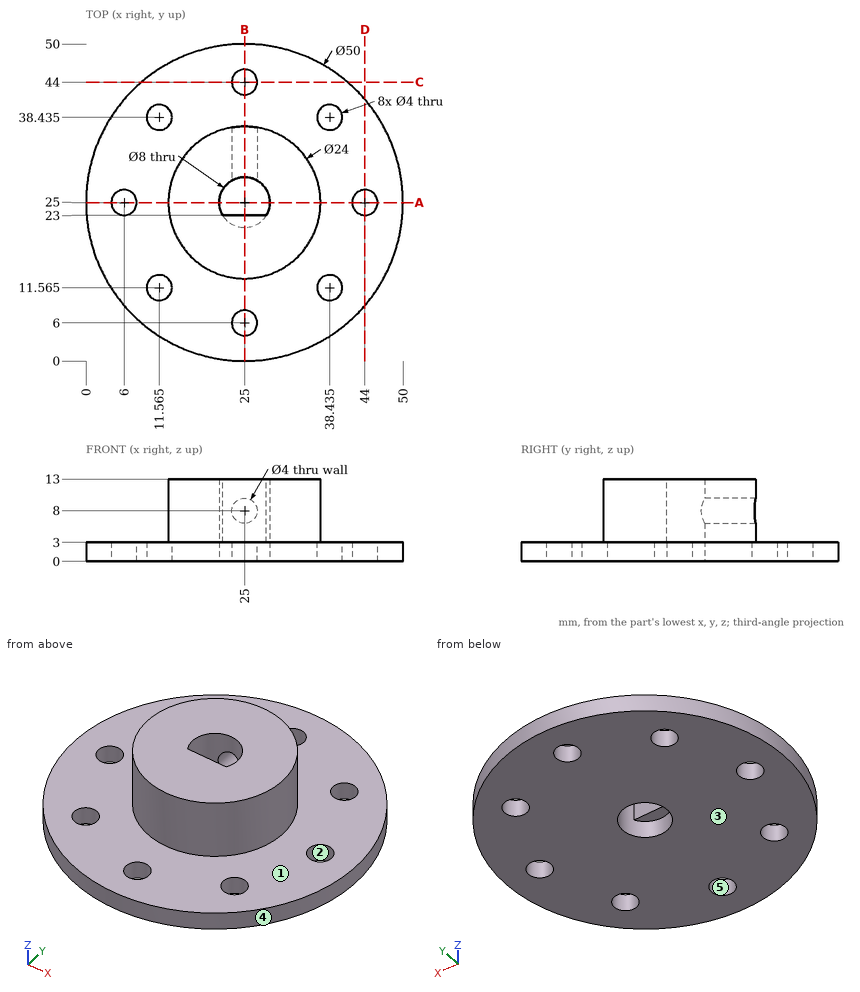
Print and shaded views of the part. All mm, measured from the part's lowest x, y and z. A direction names the side the tool comes from. Give positions to 0.01 mm unless a question says otherwise; leave off trailing zeros. Loops run counter-clockwise (first coordinate to the right, second up) from the corner with the lowest first, then second, coordinate; pieces in that order, holes last. Notation, with made-up numbers: (4, -19) -> (20, -19) arc R7 cw to (20, -6) -> close; hole circle Ø11 at (43, -23.5). An arc over 180 degrees is marked (long way). Use CSV: the item, a comma, the result in double quotes. Start each with the question number.
1) Flat gauge pins, fed straight in: pin 1 Ø6.5 at (x, y) = (25, 25) entering from +Z; pin 2 Ø0.6 at (x, y) = (26.5, 22) entering from -Z; pin 3 Ø6.5 at (x, y) = (25, 6) entering from +Z; pin 4 Ø3.5 at (x, z) = (25, 8) entering from -Y. Where does each tip first touch, or does it go through?
2) Slice it at C-C on y = 44. Give the cut face in (x, z).
3) Wall check: line 1 (Y direction, x = 25, z = 1.8); line 2 (X direction, y = 24.5, z = 0.75) (1 decimal); line 3 (Y direction, x = 24, z = 1.5). Give the ranges that are in metal, low to high.
4) Tool access for the marked faces 1 and 2: list every direction of +Z, -Z, +X, -X, +Y, -Y with a clear straight run to the whole face (end or side of a thin tool).
5) Slice it at B-B on x = 25. Give the cut face in (y, z).
6) Mould opens along X. For the marked faces 3, 4 and 5 say: released by +X, released by -X, zero draft, split by the parting line, or undercut.
7) Slice it at A-A on y = 25. Give the cut face in (x, z), plus the area to 3 significant figures.
Computed values:
1,pin 1,"stops at z = 13"
1,pin 2,"stops at z = 3"
1,pin 3,"stops at z = 3"
1,pin 4,"stops at y = 13"
2,outline,"(8.75, 0) -> (23, 0) -> (23, 3) -> (8.75, 3) -> close; (27, 0) -> (41.25, 0) -> (41.25, 3) -> (27, 3) -> close"
3,line 1,"y = 0 to 4, 8 to 21, 29 to 42, 46 to 50"
3,line 2,"x = 0 to 4.1, 7.9 to 21, 29 to 42.1, 45.9 to 50"
3,line 3,"y = 0.02 to 4.27, 7.73 to 21.13, 28.87 to 42.27, 45.73 to 49.98"
4,face 1,"+Z"
4,face 2,"+Z, -Z"
5,outline,"(0, 0) -> (4, 0) -> (4, 3) -> (0, 3) -> close; (8, 0) -> (21, 0) -> (21, 3) -> (23, 3) -> (23, 13) -> (13, 13) -> (13, 3) -> (8, 3) -> close; (29, 0) -> (42, 0) -> (42, 3) -> (37, 3) -> (37, 6) -> (29, 6) -> close; (29, 10) -> (37, 10) -> (37, 13) -> (29, 13) -> close; (46, 0) -> (50, 0) -> (50, 3) -> (46, 3) -> close"
6,face 3,"zero draft"
6,face 4,"split by the parting line"
6,face 5,"undercut"
7,outline,"(0, 0) -> (4, 0) -> (4, 3) -> (0, 3) -> close; (8, 0) -> (21, 0) -> (21, 13) -> (13, 13) -> (13, 3) -> (8, 3) -> close; (29, 0) -> (42, 0) -> (42, 3) -> (37, 3) -> (37, 13) -> (29, 13) -> close; (46, 0) -> (50, 0) -> (50, 3) -> (46, 3) -> close"
7,area,"262 mm^2"
